from build123d import *

# Parameters (mm, degrees)
SKETCH_R        = 1.55
EXTRUDE_DEPTH   = 6
SKETCH001_R     = 5
POCKET_DEPTH    = 18
FILLET_R        = 2.5
SKETCH002_R     = 3
POCKET001_DEPTH = 2


with BuildPart() as part:
    # Sketch → Extrude (new body)
    with BuildSketch(Plane.XY):
        with BuildLine():
            Line((-7, 11.429286), (-7, 6.494486))
            Line((-7, 6.494486), (-12.1, 3.55))
            Line((-12.1, 3.55), (-12.1, -3.55))
            Line((-12.1, -3.55), (-7, -6.494486))
            Line((-7, -6.494486), (-7, -11.429286))
            Line((-7, -11.429286), (7, -11.429286))
            Line((7, -11.429286), (7, -6.494486))
            Line((7, -6.494486), (12.1, -3.55))
            Line((12.1, -3.55), (12.1, 3.55))
            Line((12.1, 3.55), (7, 6.494486))
            Line((7, 6.494486), (7, 11.429286))
            ThreePointArc((-7, 11.429286), (0, 8.570714), (7, 11.429286))
        make_face()
        with Locations((-8.55, 0)):
            Circle(SKETCH_R, mode=Mode.SUBTRACT)
        with Locations((8.55, 0)):
            Circle(SKETCH_R, mode=Mode.SUBTRACT)
    extrude(amount=EXTRUDE_DEPTH)

    # Sketch001 → Pocket (cut)
    with BuildSketch(Plane.XZ.offset(11.429286)):
        with Locations((0, 6.4)):
            Circle(SKETCH001_R)
    extrude(amount=-POCKET_DEPTH, mode=Mode.SUBTRACT)

    # Fillet
    fillet_edges = [part.edges().sort_by_distance(p)[0] for p in [
        (-7, 6.494486, 3),
        (-12.1, 3.55, 3),
        (7, 6.494486, 3),
        (-12.1, -3.55, 3),
        (-7, -6.494486, 3),
        (7, -6.494486, 3),
        (12.1, -3.55, 3),
        (12.1, 3.55, 3),
    ]]
    fillet(fillet_edges, radius=FILLET_R)

    # Sketch002 → Pocket001 (cut)
    with BuildSketch(Plane(origin=(0, 0, 0), x_dir=(1, 0, 0), z_dir=(0, 0, -1))):
        with Locations((-8.55, 0)):
            Circle(SKETCH002_R)
        with Locations((8.55, 0)):
            Circle(SKETCH002_R)
    extrude(amount=-POCKET001_DEPTH, mode=Mode.SUBTRACT)


solid = part.part
Source: CAD feature listing. Evaluate the final solid. Frame: model axes, mm. A direction names the side the tool comes from. Give positions to 0.01 mm unless a question says otherwise; leave off trailing zeros. Order: outer loops, then holes, each group sorted by start corner. A loop starts at its lowest first (then second) coordinate and runs counter-clockwise, first axis right, second up. Notation, with made-up numbers: (-20, -40) -> (17, -40) arc R10 ccw to (17, -26) -> close; hole circle Ø2 at (30, 61.5). An arc over 180 degrees is marked (long way). Write item = value, one per line.
Item 1: Section query C-C (x = 8.55). Output: boundary loops of the cut face in (y, z), then the cut area to 3 significant figures.
Check result:
outline = (-5.6, 0) -> (-3, 0) -> (-3, 2) -> (-1.55, 2) -> (-1.55, 6) -> (-5.6, 6) -> close; (1.55, 2) -> (3, 2) -> (3, 0) -> (5.6, 0) -> (5.6, 6) -> (1.55, 6) -> close
area = 42.8 mm²
Item 2: Section query A-A (y = 0). Output: boundary loops of the cut face in (x, z).
Check result:
outline = (-12.1, 0) -> (-11.55, 0) -> (-11.55, 2) -> (-10.1, 2) -> (-10.1, 6) -> (-12.1, 6) -> close; (-7, 2) -> (-5.55, 2) -> (-5.55, 0) -> (5.55, 0) -> (5.55, 2) -> (7, 2) -> (7, 6) -> (4.98, 6) arc R5 cw to (-4.98, 6) -> (-7, 6) -> close; (10.1, 2) -> (11.55, 2) -> (11.55, 0) -> (12.1, 0) -> (12.1, 6) -> (10.1, 6) -> close
Item 3: Section query D-D (y = -2.5). Output: boundary loops of the cut face in (x, z).
Check result:
outline = (-12.07, 0) -> (-10.21, 0) -> (-10.21, 2) -> (-6.89, 2) -> (-6.89, 0) -> (6.89, 0) -> (6.89, 2) -> (10.21, 2) -> (10.21, 0) -> (12.07, 0) -> (12.07, 6) -> (4.98, 6) arc R5 cw to (-4.98, 6) -> (-12.07, 6) -> close
Item 4: Set-up query: faces 5 (the face through (0, 6.571, 4)), 6 (the face through (7, 10, 3)), 7 (the face through (-7, 10, 3)). Return all of +Z, -Z, +X, -X, +Y, -Y with unobstructed straight access to the full face (end or side cutting, diameter ignored); none if empty.
Check result:
face_5 = +Z, -Y
face_6 = +Z, -Z, +X, +Y
face_7 = +Z, -Z, -X, +Y
Item 5: Contact query for flat-ended pins moving along their axis: pin 1 (1 mm diameter, centred on y = -5.5, z = 1, fed in from -X); pin 2 (3 mm diameter, centred on y = -9.5, z = 3.5, fed in from +X); pin 3 (3.5 mm diameter, centred on x = 0.5, z = 2.5, fed in from -Y); pin 4 (1 mm diameter, centred on x = -0.5, y = 0.5, fed in from +Z). Output: stop coordinate, or through.
Check result:
pin_1 = -9.59
pin_2 = 7
pin_3 = -11.43
pin_4 = 1.5
Item 6: Section query B-B (z = 1.1). Output: boundary loops of the cut face in (x, y), then the cut area to 3 significant figures.
Check result:
outline = (-12.1, -2.11) arc R2.5 ccw to (-10.85, -4.27) -> (-8.25, -5.77) arc R2.5 cw to (-7, -7.94) -> (-7, -11.43) -> (7, -11.43) -> (7, -7.94) arc R2.5 cw to (8.25, -5.77) -> (10.85, -4.27) arc R2.5 ccw to (12.1, -2.11) -> (12.1, 2.11) arc R2.5 ccw to (10.85, 4.27) -> (8.25, 5.77) arc R2.5 cw to (7, 7.94) -> (7, 11.43) arc R10 cw to (-7, 11.43) -> (-7, 7.94) arc R2.5 cw to (-8.25, 5.77) -> (-10.85, 4.27) arc R2.5 ccw to (-12.1, 2.11) -> close; hole circle Ø6 at (-8.55, 0); hole circle Ø6 at (8.55, 0)
area = 338 mm²
Item 7: Ray query, probe 1 along X at (y, z) = (0, 0.35); probe 2 along X at (y, z) = (0, 4.6); probe 3 along Z at (x, y) = (-9.5, -1.75). Return the intervals inside material, ascending.
Check result:
probe_1 = -12.1 to -11.55, -5.55 to 5.55, 11.55 to 12.1
probe_2 = -12.1 to -10.1, -7 to -4.66, 4.66 to 7, 10.1 to 12.1
probe_3 = 2 to 6
Item 8: Mould query, pull axis Y, two halves, no side actions, for faces 1 (the face through (5.553, -0.132, 0.986)), 2 (the face through (-5.78, 1.15, 0.99)), 3 (the face through (11.756, 3.372, 3.042)), 4 (the face through (-0.1, -2.6, 1.4)). Classes: +Y half, -Y half, draft (parallel to the pull), parting line (faces both ways), or undercut.
Check result:
face_1 = undercut
face_2 = undercut
face_3 = +Y half
face_4 = draft
